Geometry: final body of the model. Coordinates: model frame, mm. A direction names the side the tool comes from. Coordinates: 2 decimals unless noted, no trailing zeros. Order: outer loops, then holes, each group sorted by start corner. A loop starts at its lowest first (then second) coordinate and runs counter-clockwise, first axis right, second up. Notation, with made-up numbers: M 59.25,88.5 L 64.25,88.5 A18 cw 64.25,102.5 Z; hole C 24.5,75.5 d11. An arc over 180 degrees is marked long. Use CSV: the item, a comma, the result in double quotes. Start each with the question number.
1. Section query D-D on x = -14.5. Return the cut outline in (y, z).
2. Section query A-A on x = 22.25. Return the cut outline in (y, z), and give its area (3 significant figures).
3. Material intervals for line 1 (Y direction, x = 0.5, z = 14.5); line 2 (Z direction, x = 22, y = 9); line 3 (X direction, y = 3.5, z = -19), sorted ascending.
4. Section query B-B on y = 10.25. Return the cut outline in (x, z).
5. Section query C-C on z = 14.5. Return the cut outline in (x, y), and give its area (3 significant figures).
6. Set-up query: faces 1 (the flat face through (22, 17, -20)), 2 (the flat face through (-27, 2, 27)), 3 (the cylindrical face through (23.94, 14.46, -21.59)). Return all of +Z, -Z, +X, -X, +Y, -Y with unobstructed straight access to the full face (end or side cutting, diameter ignored); none if empty.
7. First-contact query: P1, Ø2, axis at x = 20, y = 12.5, coming from the +Z side; P2, Ø1.4, axis at x = -26, z = 26.5, coming from the +Y side; P3, Ø6, axis at x = -20.5, y = 5.5, coming from the +Z side; P4, Ø10, axis at y = 11.5, z = 5.5, coming from the -X side. Flat tips, straight axial feed; report the tip coordinate or a pass-through.
from build123d import *

# Parameters (mm, degrees)
SKETCH1_W           = 55
SKETCH1_H           = 55
BOSS_EXTRUDE1_DEPTH = 2
SKETCH2_R           = 3
BOSS_EXTRUDE2_DEPTH = 10
FILLET1_R           = 2.8
SKETCH3_R           = 2.5
BOSS_EXTRUDE3_DEPTH = 5


with BuildPart() as part:
    # Sketch1 → Boss-Extrude1 (new body)
    with BuildSketch(Plane(origin=(0, 0, 0), x_dir=(1, 0, 0), z_dir=(0, 1, 0))):
        Rectangle(SKETCH1_W, SKETCH1_H)
    extrude(amount=BOSS_EXTRUDE1_DEPTH)

    # Sketch2 → Boss-Extrude2 (add)
    with BuildSketch(Plane(origin=(0, 2, 0), x_dir=(1, 0, 0), z_dir=(0, 1, 0))):
        with Locations(Location((-22.25, -22.25, 0), (0, 0, 270))):
            Circle(SKETCH2_R)
        with Locations(Location((22.25, 19.75, 0), (0, 0, 270))):
            Circle(SKETCH2_R)
    extrude(amount=BOSS_EXTRUDE2_DEPTH)

    # Fillet1
    fillet1_edges = [part.edges().sort_by_distance(p)[0] for p in [
        (-22.25, 2, 19.25),
        (22.25, 2, -22.75),
    ]]
    fillet(fillet1_edges, radius=FILLET1_R)

    # Sketch3 → Boss-Extrude3 (add)
    with BuildSketch(Plane(origin=(0, 12, 0), x_dir=(1, 0, 0), z_dir=(0, 1, 0))):
        with Locations(Location((-22.25, -22.25, 0), (0, 0, 270))):
            Circle(SKETCH3_R)
        with Locations(Location((22.25, 19.75, 0), (0, 0, 270))):
            Circle(SKETCH3_R)
    extrude(amount=BOSS_EXTRUDE3_DEPTH)


solid = part.part
Results list:
1,outline,"M 0,-27.5 L 2,-27.5 L 2,27.5 L 0,27.5 Z"
2,outline,"M 0,-27.5 L 2,-27.5 L 2,-25.55 A2.8 cw 4.8,-22.75 L 12,-22.75 L 12,-22.25 L 17,-22.25 L 17,-17.25 L 12,-17.25 L 12,-16.75 L 4.8,-16.75 A2.8 cw 2,-13.95 L 2,27.5 L 0,27.5 Z"
2,area,"198 mm²"
3,line 1,"y = 0 to 2"
3,line 2,"z = -22.74 to -16.76"
3,line 3,"x = 19.02 to 25.47"
4,outline,"C -22.25,22.25 d6; C 22.25,-19.75 d6"
5,outline,"M -27.5,0 L 27.5,0 L 27.5,2 L -27.5,2 Z"
5,area,"110 mm²"
6,face 1,"+Z, -Z, +X, -X, +Y"
6,face 2,"+Z, -X, +Y"
6,face 3,"+Y"
7,P1,"stops at z = -17.09"
7,P2,"stops at y = 2.13"
7,P3,"stops at z = 26.18"
7,P4,"passes through"
